Check sheet for the modelled part. Datum: model origin and axes. Units: mm. Round coordinates to 2 decimals unless told otherwise and drop trailing zeros. Loops run counter-clockwise (first coordinate to the right, second up) from the corner with the lowest first, then second, coordinate; pieces in that order, holes last. Notation, with made-up numbers: (-17.5, -3.75) - (-0.5, -3.75) arc R30 cw to (-0.5, 20.25) - close; hole circle Ø8 at (7, -12). An arc over 180 degrees is marked (long way). Put each result on its own line as item: value. Start each with the question number.
Item 1: Draft check along X on faces 1 (the cylindrical face through (19.89, -18.24, 9.39)), 2 (the flat face through (1.894, 20.095, 9.392)), 3 (the cylindrical face through (-9.1, -15.79, 9.39)). Enter one of: pulls with the +X half, pulls with the -X half, needs draft (parallel to the pull), parting line crosses it, or undercut.
Item 2: Material ranges on line 1 along Y through (x, z) = (18.5, 16.75); line 2 along Y through (x, z) = (-17, 11); line 3 along Y through (x, z) = (-20.5, 1.75), recorded low to high.
Item 3: Gauge pin test, flat ends, axial feed: pin 1 Ø1 at (y, z) = (-12.5, 11.5) entering from +X; pin 2 Ø3 at (y, z) = (8, 4) entering from -X; pin 3 Ø1 at (y, z) = (-21, 17) entering from +X. Record the tip position at first contact, or that the pin passes through.
Item 4: Section check C-C, the plane x = 24.5. Record the cut outline in (y, z).
from build123d import *

# Parameters (mm, degrees)
MODEL_R             = 26.9875
BOSS_EXTRUDE1_DEPTH = 19.05


with BuildPart() as part:
    # Model → Boss-Extrude1 (new body)
    with BuildSketch(Plane.XY):
        with Locations(Location((0, 0, 0), (0, 0, 180))):
            Circle(MODEL_R)
        with BuildLine():
            Line((-8.070485832, 16.757663602), (-8.754511726, 19.987689799))
            ThreePointArc((-8.754511726, 19.987689799), (-8.707484905, 20.324784918), (-8.455586843, 20.553677922))
            ThreePointArc((-8.455586843, 20.553677922), (-5.752253282, 21.467701488), (-2.95408596, 22.027800642))
            ThreePointArc((-2.95408596, 22.027800642), (-2.621489336, 21.955522516), (-2.412215355, 21.687102989))
            Line((-2.412215355, 21.687102989), (-1.38958606, 18.5478053))
            ThreePointArc((-1.38958606, 18.5478053), (-1.197947162, 18.291000428), (-0.889763559, 18.203267447))
            ThreePointArc((-0.889763559, 18.203267447), (-4e-09, 18.224999999), (0.88976355, 18.203267448))
            ThreePointArc((0.88976355, 18.203267448), (1.197947153, 18.291000429), (1.38958605, 18.547805301))
            Line((1.38958605, 18.547805301), (2.412215346, 21.68710299))
            ThreePointArc((2.412215346, 21.68710299), (2.621489327, 21.955522516), (2.954085951, 22.027800641))
            ThreePointArc((2.954085951, 22.027800641), (5.752253273, 21.467701488), (8.455586835, 20.553677923))
            ThreePointArc((8.455586835, 20.553677923), (8.707484897, 20.324784919), (8.754511717, 19.9876898))
            Line((8.754511717, 19.9876898), (8.070485823, 16.757663603))
            ThreePointArc((8.070485823, 16.757663603), (8.108047539, 16.439444611), (8.331075878, 16.209373819))
            ThreePointArc((8.331075878, 16.209373819), (9.112499995, 15.783312983), (9.872191562, 15.319610264))
            ThreePointArc((9.872191562, 15.319610264), (10.182952881, 15.241497453), (10.47731947, 15.368077548))
            Line((10.47731947, 15.368077548), (12.932591265, 17.575474446))
            ThreePointArc((12.932591265, 17.575474446), (13.248037611, 17.703295585), (13.572213798, 17.599591967))
            ThreePointArc((13.572213798, 17.599591967), (15.715448207, 15.71544821), (17.599591964, 13.572213802))
            ThreePointArc((17.599591964, 13.572213802), (17.703295582, 13.248037614), (17.575474443, 12.932591268))
            Line((17.575474443, 12.932591268), (15.368077544, 10.477319473))
            ThreePointArc((15.368077544, 10.477319473), (15.24149745, 10.182952884), (15.319610261, 9.872191565))
            ThreePointArc((15.319610261, 9.872191565), (15.78331298, 9.112499998), (16.209373816, 8.331075881))
            ThreePointArc((16.209373816, 8.331075881), (16.439444608, 8.108047543), (16.7576636, 8.070485826))
            Line((16.7576636, 8.070485826), (19.987689797, 8.75451172))
            ThreePointArc((19.987689797, 8.75451172), (20.324784916, 8.707484899), (20.55367792, 8.455586837))
            ThreePointArc((20.55367792, 8.455586837), (21.467701485, 5.752253275), (22.027800638, 2.954085954))
            ThreePointArc((22.027800638, 2.954085954), (21.955522513, 2.62148933), (21.687102986, 2.412215349))
            Line((21.687102986, 2.412215349), (18.547805297, 1.389586053))
            ThreePointArc((18.547805297, 1.389586053), (18.291000425, 1.197947156), (18.203267445, 0.889763553))
            ThreePointArc((18.203267445, 0.889763553), (18.224999996, -2e-09), (18.203267445, -0.889763556))
            ThreePointArc((18.203267445, -0.889763556), (18.291000425, -1.19794716), (18.547805298, -1.389586057))
            Line((18.547805298, -1.389586057), (21.687102987, -2.412215353))
            ThreePointArc((21.687102987, -2.412215353), (21.955522514, -2.621489333), (22.027800639, -2.954085957))
            ThreePointArc((22.027800639, -2.954085957), (21.467701485, -5.752253279), (20.55367792, -8.455586841))
            ThreePointArc((20.55367792, -8.455586841), (20.324784915, -8.707484903), (19.987689796, -8.754511723))
            Line((19.987689796, -8.754511723), (16.757663599, -8.070485829))
            ThreePointArc((16.757663599, -8.070485829), (16.439444608, -8.108047546), (16.209373816, -8.331075885))
            ThreePointArc((16.209373816, -8.331075885), (15.78331298, -9.112500002), (15.319610261, -9.872191568))
            ThreePointArc((15.319610261, -9.872191568), (15.24149745, -10.182952888), (15.368077545, -10.477319476))
            Line((15.368077545, -10.477319476), (17.575474443, -12.932591272))
            ThreePointArc((17.575474443, -12.932591272), (17.703295583, -13.248037618), (17.599591965, -13.572213805))
            ThreePointArc((17.599591965, -13.572213805), (15.715448207, -15.715448213), (13.572213799, -17.59959197))
            ThreePointArc((13.572213799, -17.59959197), (13.248037611, -17.703295588), (12.932591265, -17.575474449))
            Line((12.932591265, -17.575474449), (10.47731947, -15.368077551))
            ThreePointArc((10.47731947, -15.368077551), (10.182952881, -15.241497457), (9.872191562, -15.319610268))
            ThreePointArc((9.872191562, -15.319610268), (9.112499996, -15.783312986), (8.331075878, -16.209373822))
            ThreePointArc((8.331075878, -16.209373822), (8.108047539, -16.439444614), (8.070485823, -16.757663607))
            Line((8.070485823, -16.757663607), (8.754511717, -19.987689803))
            ThreePointArc((8.754511717, -19.987689803), (8.707484897, -20.324784922), (8.455586834, -20.553677926))
            ThreePointArc((8.455586834, -20.553677926), (5.752253273, -21.467701491), (2.954085951, -22.027800644))
            ThreePointArc((2.954085951, -22.027800644), (2.621489325, -21.955522517), (2.412215346, -21.687102985))
            Line((2.412215346, -21.687102985), (1.38958605, -18.547805297))
            ThreePointArc((1.38958605, -18.547805297), (1.197947153, -18.291000425), (0.889763549, -18.203267444))
            ThreePointArc((0.889763549, -18.203267444), (-4e-09, -18.224999995), (-0.889763558, -18.203267444))
            ThreePointArc((-0.889763558, -18.203267444), (-1.197947162, -18.291000425), (-1.389586059, -18.547805297))
            Line((-1.389586059, -18.547805297), (-2.412215354, -21.687102986))
            ThreePointArc((-2.412215354, -21.687102986), (-2.621489335, -21.955522513), (-2.954085959, -22.027800639))
            ThreePointArc((-2.954085959, -22.027800639), (-5.75225328, -21.467701485), (-8.455586841, -20.55367792))
            ThreePointArc((-8.455586841, -20.55367792), (-8.707484903, -20.324784915), (-8.754511723, -19.987689797))
            Line((-8.754511723, -19.987689797), (-8.070485829, -16.7576636))
            ThreePointArc((-8.070485829, -16.7576636), (-8.108047546, -16.439444608), (-8.331075884, -16.209373816))
            ThreePointArc((-8.331075884, -16.209373816), (-9.112500001, -15.78331298), (-9.872191567, -15.319610262))
            ThreePointArc((-9.872191567, -15.319610262), (-10.182952886, -15.241497451), (-10.477319475, -15.368077546))
            Line((-10.477319475, -15.368077546), (-12.93259127, -17.575474444))
            ThreePointArc((-12.93259127, -17.575474444), (-13.248037616, -17.703295583), (-13.572213803, -17.599591965))
            ThreePointArc((-13.572213803, -17.599591965), (-15.715448211, -15.715448209), (-17.599591967, -13.572213801))
            ThreePointArc((-17.599591967, -13.572213801), (-17.703295585, -13.248037614), (-17.575474446, -12.932591267))
            Line((-17.575474446, -12.932591267), (-15.368077548, -10.477319472))
            ThreePointArc((-15.368077548, -10.477319472), (-15.241497453, -10.182952883), (-15.319610265, -9.872191564))
            ThreePointArc((-15.319610265, -9.872191564), (-15.783312983, -9.112499999), (-16.209373818, -8.331075882))
            ThreePointArc((-16.209373818, -8.331075882), (-16.439444611, -8.108047543), (-16.757663603, -8.070485827))
            Line((-16.757663603, -8.070485827), (-19.9876898, -8.754511721))
            ThreePointArc((-19.9876898, -8.754511721), (-20.324784919, -8.7074849), (-20.553677923, -8.455586838))
            ThreePointArc((-20.553677923, -8.455586838), (-21.467701487, -5.752253277), (-22.027800641, -2.954085957))
            ThreePointArc((-22.027800641, -2.954085957), (-21.955522516, -2.621489333), (-21.687102989, -2.412215352))
            Line((-21.687102989, -2.412215352), (-18.5478053, -1.389586056))
            ThreePointArc((-18.5478053, -1.389586056), (-18.291000428, -1.197947159), (-18.203267448, -0.889763556))
            ThreePointArc((-18.203267448, -0.889763556), (-18.224999999, -2e-09), (-18.203267448, 0.889763552))
            ThreePointArc((-18.203267448, 0.889763552), (-18.291000429, 1.197947155), (-18.547805301, 1.389586052))
            Line((-18.547805301, 1.389586052), (-21.68710299, 2.412215348))
            ThreePointArc((-21.68710299, 2.412215348), (-21.955522518, 2.621489329), (-22.027800643, 2.954085953))
            ThreePointArc((-22.027800643, 2.954085953), (-21.46770149, 5.752253274), (-20.553677925, 8.455586836))
            ThreePointArc((-20.553677925, 8.455586836), (-20.324784921, 8.707484898), (-19.987689802, 8.754511718))
            Line((-19.987689802, 8.754511718), (-16.757663605, 8.070485824))
            ThreePointArc((-16.757663605, 8.070485824), (-16.439444614, 8.108047541), (-16.209373822, 8.331075879))
            ThreePointArc((-16.209373822, 8.331075879), (-15.783312986, 9.112499997), (-15.319610268, 9.872191563))
            ThreePointArc((-15.319610268, 9.872191563), (-15.241497457, 10.182952882), (-15.368077552, 10.477319471))
            Line((-15.368077552, 10.477319471), (-17.57547445, 12.932591266))
            ThreePointArc((-17.57547445, 12.932591266), (-17.703295589, 13.248037612), (-17.599591971, 13.572213799))
            ThreePointArc((-17.599591971, 13.572213799), (-15.715448215, 15.715448208), (-13.572213807, 17.599591965))
            ThreePointArc((-13.572213807, 17.599591965), (-13.24803762, 17.703295583), (-12.932591273, 17.575474444))
            Line((-12.932591273, 17.575474444), (-10.477319478, 15.368077546))
            ThreePointArc((-10.477319478, 15.368077546), (-10.182952889, 15.241497452), (-9.87219157, 15.319610263))
            ThreePointArc((-9.87219157, 15.319610263), (-9.112500004, 15.783312982), (-8.331075887, 16.209373818))
            ThreePointArc((-8.331075887, 16.209373818), (-8.108047548, 16.43944461), (-8.070485832, 16.757663602))
        make_face(mode=Mode.SUBTRACT)
    extrude(amount=BOSS_EXTRUDE1_DEPTH)


solid = part.part
Check result:
1. face 1: parting line crosses it
1. face 2: undercut
1. face 3: undercut
2. line 1: -19.65 to -8.44, -1.37 to 1.37, 8.44 to 19.65
2. line 2: -20.96 to -14.32, -12.29 to -8.12, 8.12 to 12.29, 14.32 to 20.96
2. line 3: -17.55 to -8.55, -2.03 to 2.03, 8.55 to 17.55
3. pin 1: x = 24.17
3. pin 2: x = -26.19
3. pin 3: x = 17.55
4. outline: (-11.32, 0) - (11.32, 0) - (11.32, 19.05) - (-11.32, 19.05) - close
